Verification items for the finished model (mm, model axes). Face numbers are marked on the shaded views. Coordinates: 2 decimals unless noted, no trailing zeros. Write each loop counter-clockwise with the first axis right and the second up, starting at its lowest first coordinate (ties: lowest second). Pieces come first, ordered by that corner, then holes. Notation, with made-up numbers: (-4, 79) -> (53, 79) arc R16 cw to (53, 92) -> close; hole circle Ø4 at (28, 72.25). An arc over 180 degrees is marked (long way). Write item = value, one per line. Start each with the question number.
(1) Material ranges on probe 1 along Y at (x, z) = (0, 3); probe 2 along Y at (x, z) = (0, 17.25); probe 3 along Z at (x, y) = (9, -4.5), recorded low to high. Write a range as [from, to].
(2) Mould release check, pull along X, two halves, no side actions. Record for the marked faces 1, 2, 3 and 4: released by +X, released by -X, zero draft, split by the parting line, or undercut.
(3) Section check C-C (z = 34.5). Record the cut outline in (x, y).
(4) Section check A-A (y = 0). Record the cut outline in (x, z), plus the area to 3 significant figures.
(5) Gauge pin test, flat ends, axial feed: pin 1 Ø1.5 at (y, z) = (-17.5, 4.5) entering from +X; pin 2 Ø3 at (y, z) = (-12.5, 8) entering from +X; pin 3 Ø1.5 at (y, z) = (-18, 5) entering from -X. Record the tip position at first contact, or that the pin passes through.
```python
from build123d import *

# Parameters (mm, degrees)
SKETCH1_R           = 19.5
BOSS_EXTRUDE1_DEPTH = 37
SHELL1_T            = -2
SKETCH2_R           = 17.5
SKETCH2_R_2         = 17.1
BOSS_EXTRUDE2_DEPTH = 2
CUT_EXTRUDE1_START  = -4
SKETCH3_R           = 19.5
CUT_EXTRUDE1_DEPTH  = 4


with BuildPart() as part:
    # Sketch1 → Boss-Extrude1 (new body)
    with BuildSketch(Plane.XY):
        Circle(SKETCH1_R)
    extrude(amount=BOSS_EXTRUDE1_DEPTH)

    # Shell1
    shell1_openings = [part.faces().sort_by_distance(p)[0] for p in [
        (0, 0, 37),
    ]]
    offset(amount=SHELL1_T, openings=shell1_openings, kind=Kind.INTERSECTION)

    # Sketch2 → Boss-Extrude2 (add)
    with BuildSketch(Plane.XY.offset(2)):
        Circle(SKETCH2_R)
        Circle(SKETCH2_R_2, mode=Mode.SUBTRACT)
    extrude(amount=BOSS_EXTRUDE2_DEPTH)

    # Sketch3 → Cut-Extrude1 (cut)
    with BuildSketch(Plane.XY.offset(37).offset(CUT_EXTRUDE1_START)):
        Circle(SKETCH3_R)
    extrude(amount=CUT_EXTRUDE1_DEPTH, mode=Mode.SUBTRACT)

    # Sketch4 → Revolve1 (revolve)
    with BuildSketch(Plane(origin=(0, 0, 0), x_dir=(1, 0, 0), z_dir=(0, 1, 0)), mode=Mode.PRIVATE) as revolve1_sk:
        Polygon((19.5, -33), (22.964101615, -39), (20.964101615, -39), (17.5, -33), align=None)
    revolve(revolve1_sk.sketch.rotate(Axis((0, 0, 33), (0, 0, 1)), 180), axis=Axis((0, 0, 33), (0, 0, 1)))


solid = part.part
```
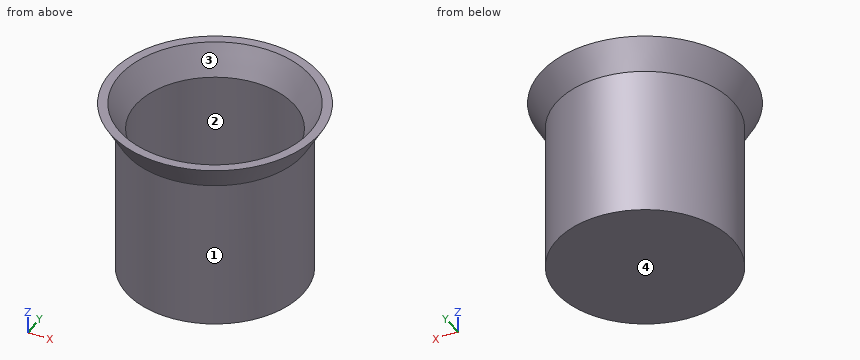
Response:
q1.probe_1 = [-19.5, -17.1], [17.1, 19.5]
q1.probe_2 = [-19.5, -17.5], [17.5, 19.5]
q1.probe_3 = [0, 2]
q2.face_1 = split by the parting line
q2.face_2 = undercut
q2.face_3 = undercut
q2.face_4 = zero draft
q3.outline = circle Ø40.73 at (0, 0); hole circle Ø36.73 at (0, 0)
q4.outline = (-22.96, 39) -> (-19.5, 33) -> (-19.5, 0) -> (19.5, 0) -> (19.5, 33) -> (22.96, 39) -> (20.96, 39) -> (17.5, 33) -> (17.5, 4) -> (17.1, 4) -> (17.1, 2) -> (-17.1, 2) -> (-17.1, 4) -> (-17.5, 4) -> (-17.5, 33) -> (-20.96, 39) -> close
q4.area = 228 mm2
q5.pin_1 = 9.98
q5.pin_2 = 16.1
q5.pin_3 = -9.09
